```python
from build123d import *

# Parameters (mm, degrees)
F1_DEPTH       = 19.5
F2_R           = 2.6
F3_DEPTH       = 17.501
F5_D           = 3.3
F5_CBORE_D     = 6.5
F5_CBORE_DEPTH = 3
F6_R           = 6
F7_SIZE        = 1


with BuildPart() as f1:
    # F0 (on Top) → F1 (new body)
    with BuildSketch(Plane.XY):
        Polygon((-22, 0), (0, 0), (0, 17.5), (-22, 17.5), (-22, 13.75), (-6, 13.75), (-6, 3.75), (-22, 3.75), align=None)
    extrude(amount=F1_DEPTH)

    # F2 (on face) → F3 (cut, through all)
    with BuildSketch(Plane(origin=(0, 17.5, 0), x_dir=(-1, 0, 0), z_dir=(0, 1, 0))):
        with Locations((16, 9.75)):
            Circle(F2_R)
    extrude(amount=-F3_DEPTH, mode=Mode.SUBTRACT)

    # F5 (through all)
    with Locations(Plane(origin=(-6, 0, 0), x_dir=(0, -1, 0), z_dir=(-1, 0, 0))):
        with Locations((-8.75, 9.75)):
            CounterBoreHole(F5_D / 2, F5_CBORE_D / 2, F5_CBORE_DEPTH)

    # F6
    f6_edges = [f1.edges().sort_by_distance(p)[0] for p in [
        (-22, 15.625, 0),
        (-22, 15.625, 19.5),
        (-22, 1.875, 19.5),
        (-22, 1.875, 0),
    ]]
    fillet(f6_edges, radius=F6_R)

    # F7
    f7_edges = [f1.edges().sort_by_distance(p)[0] for p in [
        (-8, 17.5, 0),
        (-8, 0, 0),
        (-11, 3.75, 0),
        (-11, 13.75, 0),
    ]]
    chamfer(f7_edges, length=F7_SIZE)


solid = f1.part
```
Verification items for the finished model (mm, model axes). A direction names the side the tool comes from. Round coordinates to 2 decimals unless told otherwise and drop trailing zeros. Order: outer loops, then holes, each group sorted by start corner. A loop starts at its lowest first (then second) coordinate and runs counter-clockwise, first axis right, second up. Notation, with made-up numbers: (21, 79.25) -> (44, 79.25) arc R13 ccw to (44, 93.25) -> close; hole circle Ø9 at (-11.75, 76.25). An arc over 180 degrees is marked (long way). Put each result on its own line as item: value. Start each with the question number.
(1) Section check A-A (y = 8.75). Enter the section's corners in (x, z), then the cut area to 3 significant figures.
(2) Tool access check on faces 4 (the face through (-4.521, 11.145, 11.947)), 5 (the face through (-11.07, 3.26, 18.99)), 6 (the face through (-21.49, 3.26, 9.7)), 7 (the face through (-11.07, 14.24, 0.51)). Record the directions out of +Z, -Z, +X, -X, +Y, -Y that give a thin tool (end or side, any length) a straight path to the whole face; none if there is none.
(3) Draft check along Z on faces 1 (the face through (-21.5, 17, 9.7)), 2 (the face through (-19.686, 14.021, 17.268)), 3 (the face through (-1.48, 7.44, 8.75)). Enter one of: +Z half, -Z half, draft (parallel to the pull), parting line (faces both ways), or undercut.
(4) Section check D-D (y = 15.75). Enter the section's corners in (x, z), then the cut area to 3 significant figures.
(5) Section check B-B (z = 9.75). Enter the section's corners in (x, y).
(6) Depth check by flat-ended pin: pin 1 Ø5 at (y, z) = (8.5, 10.5) entering from -X; pin 2 Ø4 at (x, z) = (-16, 9.75) entering from +Y; pin 3 Ø3.5 at (y, z) = (10, 10) entering from -X. Enter the tip coordinate at first touch or a pass-through.
(7) Section check C-C (x = -7.25). Enter the section's corners in (y, z).
(8) Material ranges on line 1 along Y through (x, z) = (-18.75, 14.5); line 2 along Z through (x, y) = (-4.15, 8.75), recorded low to high.
Completed:
1. outline: (-6, 0) -> (0, 0) -> (0, 8.1) -> (-3, 8.1) -> (-3, 6.5) -> (-6, 6.5) -> close; (-6, 13) -> (-3, 13) -> (-3, 11.4) -> (0, 11.4) -> (0, 19.5) -> (-6, 19.5) -> close
1. area: 87.6 mm2
2. face 4: -X
2. face 5: +Z, -X
2. face 6: +Z, -Z, -X
2. face 7: -Z, -X
3. face 1: draft
3. face 2: +Z half
3. face 3: undercut
4. outline: (-22, 6) arc R6 ccw to (-16, 0) -> (0, 0) -> (0, 19.5) -> (-16, 19.5) arc R6 ccw to (-22, 13.5) -> close; hole circle Ø5.2 at (-16, 9.75)
4. area: 392 mm2
5. outline: (-22, 1) -> (-21, 0) -> (-18.6, 0) -> (-18.6, 3.75) -> (-21, 3.75) -> (-22, 2.75) -> close; (-22, 14.75) -> (-21, 13.75) -> (-18.6, 13.75) -> (-18.6, 17.5) -> (-21, 17.5) -> (-22, 16.5) -> close; (-13.4, 0) -> (0, 0) -> (0, 7.1) -> (-3, 7.1) -> (-3, 5.5) -> (-6, 5.5) -> (-6, 3.75) -> (-13.4, 3.75) -> close; (-13.4, 13.75) -> (-6, 13.75) -> (-6, 12) -> (-3, 12) -> (-3, 10.4) -> (0, 10.4) -> (0, 17.5) -> (-13.4, 17.5) -> close
6. pin 1: stops at x = -6
6. pin 2: passes through
6. pin 3: stops at x = -3
7. outline: (0, 1) -> (1, 0) -> (2.75, 0) -> (3.75, 1) -> (3.75, 18.5) -> (2.75, 19.5) -> (1, 19.5) -> (0, 18.5) -> close; (13.75, 1) -> (14.75, 0) -> (16.5, 0) -> (17.5, 1) -> (17.5, 18.5) -> (16.5, 19.5) -> (14.75, 19.5) -> (13.75, 18.5) -> close
8. line 1: y = 0 to 3.75, 13.75 to 17.5
8. line 2: z = 0 to 6.5, 13 to 19.5
